Source: CAD feature listing. Evaluate the final solid. Frame: model axes, mm. A direction names the side the tool comes from. Round coordinates to 2 decimals unless told otherwise and drop trailing zeros. Write each loop counter-clockwise with the first axis right and the second up, starting at its lowest first coordinate (ties: lowest second). Pieces come first, ordered by that corner, then holes. Notation, with made-up numbers: M 71,64 L 89,64 A23 ccw 89,87 Z; hole C -12.75,-29 d3. An arc over 180 degrees is marked long. Answer in a Markdown table with one row per item.
from build123d import *

# Parameters (mm, degrees)
F1_DEPTH = 25.4
F3_DEPTH = 25.4
F5_DEPTH = 25.4


with BuildPart() as f1:
    # F0 (on Top) → F1 (new body)
    with BuildSketch(Plane.XY):
        with BuildLine():
            ThreePointArc((-49.171314, 59.99193), (-55.475723, 59.232373), (-57.970132, 53.392816))
            Line((-57.970132, 53.392816), (-45.007356, -54.199724))
            ThreePointArc((-45.007356, -54.199724), (-42.915981, -58.191256), (-38.702947, -59.790168))
            Line((-38.702947, -59.790168), (49.316182, -59.790168))
            ThreePointArc((49.316182, -59.790168), (53.80631, -57.930296), (55.666182, -53.440168))
            Line((55.666182, -53.440168), (55.666182, 11.017219))
            ThreePointArc((55.666182, 11.017219), (54.615333, 14.516005), (51.810591, 16.856776))
            Line((51.810591, 16.856776), (-49.171314, 59.99193))
        make_face()
    extrude(amount=F1_DEPTH)

    # F2 (on face) → F3 (cut, through all)
    with BuildSketch(Plane.XY.offset(25.4)):
        with BuildLine():
            Line((33.666182, -7.790168), (-24.333818, -7.790168))
            ThreePointArc((-24.333818, -7.790168), (-31.404886, -10.7191), (-34.333818, -17.790168))
            Line((-34.333818, -17.790168), (-34.333818, -37.790168))
            ThreePointArc((-34.333818, -37.790168), (-31.404886, -44.861235), (-24.333818, -47.790168))
            Line((-24.333818, -47.790168), (33.666182, -47.790168))
            ThreePointArc((33.666182, -47.790168), (40.73725, -44.861235), (43.666182, -37.790168))
            Line((43.666182, -37.790168), (43.666182, -17.790168))
            ThreePointArc((43.666182, -17.790168), (40.73725, -10.7191), (33.666182, -7.790168))
        make_face()
    extrude(amount=-F3_DEPTH, mode=Mode.SUBTRACT)

    # F4 (on face) → F5 (cut, through all)
    with BuildSketch(Plane.XY.offset(25.4)):
        with BuildLine():
            Line((-34.637267, 4.209832), (21.548996, 4.209832))
            ThreePointArc((21.548996, 4.209832), (27.427183, 9.00695), (23.905918, 15.727524))
            Line((23.905918, 15.727524), (-35.328801, 41.030064))
            ThreePointArc((-35.328801, 41.030064), (-41.285723, 40.312373), (-43.642645, 34.794681))
            Line((-43.642645, 34.794681), (-40.594189, 9.492141))
            ThreePointArc((-40.594189, 9.492141), (-38.618087, 5.720615), (-34.637267, 4.209832))
        make_face()
    extrude(amount=-F5_DEPTH, mode=Mode.SUBTRACT)


solid = f1.part
Q1. Section D-D (x = 36). Return loops of the section in (y, z).
Solutions:
| item | result |
|---|---|
| outline | M -59.79,0 L -47.51,0 L -47.51,25.4 L -59.79,25.4 Z; M -8.07,0 L 23.61,0 L 23.61,25.4 L -8.07,25.4 Z |
Q2. Material intervals for probe 1 along Y at (x, z) = (-4, 11.25); probe 2 along Y at (x, z) = (24.5, 3); probe 3 along X at (y, z) = (21, 16.75), sorted ascending.
Solutions:
| item | result |
|---|---|
| probe 1 | y = -59.79 to -47.79, -7.79 to 4.21, 27.65 to 40.7 |
| probe 2 | y = -59.79 to -47.79, -7.79 to 4.99, 15.43 to 28.52 |
| probe 3 | x = -54.07 to -41.98, 11.56 to 42.11 |
Q3. Pull-direction query (Y, two-part tool) for faces 3 (the flat face through (-7, 4.21, 13)), 4 (the flat face through (5, -59.79, 13)), 5 (the flat face through (55.666, -22, 13)); classes: pulls with the +Y half, pulls with the -Y half, needs draft (parallel to the pull), parting line crosses it, or undercut.
Solutions:
| item | result |
|---|---|
| face 3 | undercut |
| face 4 | pulls with the -Y half |
| face 5 | needs draft |
Q4. Section A-A (y = -45). Return loops of the section in (x, z), and give its area (3 significant figures).
Solutions:
| item | result |
|---|---|
| outline | M -46.12,0 L -31.26,0 L -31.26,25.4 L -46.12,25.4 Z; M 40.6,0 L 55.67,0 L 55.67,25.4 L 40.6,25.4 Z |
| area | 760 mm2 |
Q5. Access query for faces 1 (the flat face through (4, -47.79, 13)), 2 (the flat face through (-2, 1, 0)). Directions: +Z, -Z, +X, -X, +Y, -Y. A direction counts if a zero-diameter tool reaches every point of the face in a straight line with its end or side. Return the directions, or none.
Solutions:
| item | result |
|---|---|
| face 1 | +Z, -Z |
| face 2 | -Z, +X, -X, +Y, -Y |
Q6. Section C-C (z = 10.25). Return loops of the section in (x, y), and give its area (3 significant figures).
Solutions:
| item | result |
|---|---|
| outline | M -57.97,53.39 L -45.01,-54.2 A6.35 ccw -38.7,-59.79 L 49.32,-59.79 A6.35 ccw 55.67,-53.44 L 55.67,11.02 A6.35 ccw 51.81,16.86 L -49.17,59.99 A6.35 ccw Z; hole M -43.64,34.79 L -40.59,9.49 A6 ccw -34.64,4.21 L 21.55,4.21 A6 ccw 23.91,15.73 L -35.33,41.03 A6 ccw Z; hole M -34.33,-37.79 A10 ccw -24.33,-47.79 L 33.67,-47.79 A10 ccw 43.67,-37.79 L 43.67,-17.79 A10 ccw 33.67,-7.79 L -24.33,-7.79 A10 ccw -34.33,-17.79 Z |
| area | 5,740 mm2 |
Q7. Section B-B (x = -28). Return loops of the section in (y, z), and give its area (3 significant figures).
Solutions:
| item | result |
|---|---|
| outline | M -59.79,0 L -47.09,0 L -47.09,25.4 L -59.79,25.4 Z; M -8.49,0 L 4.21,0 L 4.21,25.4 L -8.49,25.4 Z; M 37.9,0 L 50.95,0 L 50.95,25.4 L 37.9,25.4 Z |
| area | 976 mm2 |
Q8. Contact query for flat-ended pins moving along their axis: pin 1 Ø12 at (y, z) = (38, 19) entering from -X; pin 2 Ø1.5 at (x, z) = (-10.5, 2.5) entering from +Y; pin 3 Ø12 at (y, z) = (-40.5, 14.5) entering from -X. Output: stop coordinate, or through.
Solutions:
| item | result |
|---|---|
| pin 1 | stops at x = -56.84 |
| pin 2 | stops at y = 43.79 |
| pin 3 | stops at x = -47.38 |
